Part model, mm, in its own coordinate system. Coordinates: 2 decimals unless noted, no trailing zeros. Loops run counter-clockwise (first coordinate to the right, second up) from the corner with the lowest first, then second, coordinate; pieces in that order, holes last. Notation, with made-up numbers: M 36,25.5 L 58,25.5 A25 ccw 58,46.5 Z; hole C 19.5,70.25 d4. An arc over 180 degrees is marked long. Use a Markdown table: item, result. Add a question column.
1) Wall check: probe 1 along Y at (x, z) = (6.45, 2.75); probe 2 along Y at (x, z) = (5.7, 5); probe 3 along Z at (x, y) = (6.65, -2.5). Give the ranges that are in metal, low to high. Write a range as from..to.
2) Band-saw the part on A-A (z = 9). List the corners of the cut face in (x, y), plus the area to 3 significant figures.
3) Pull direction Y, two halves, no side cores. Call faces 1 (the cylindrical face through (6.089, -6.579, 0.285)), 2 (the flat face through (8, 0, 0)), 3 (the cylindrical face through (4.68, 5.44, 5.57)): released by +Y, released by -Y, zero draft, split by the parting line, or undercut.
4) Pin check, flat tip, straight feed: pin 1 Ø1 at (x, z) = (9, 2) entering from -Y. Stop position of the tip, or through.
from build123d import *

# Parameters (mm, degrees)
BOSS_EXTRUDE1_DEPTH = 11
FILLET1_R           = 1
FILLET2_R           = 1
FILLET3_R           = 0.25


with BuildPart() as part:
    # Sketch1 → Boss-Extrude1 (new body)
    with BuildSketch(Plane.XY):
        with BuildLine():
            Line((6.738137725, -6.88), (4.878137725, -6.88))
            Line((4.878137725, -6.88), (4.531835438, -5.38))
            ThreePointArc((4.531835438, -5.38), (7.034339517, 0), (4.531835438, 5.38))
            Line((4.531835438, 5.38), (4.878137725, 6.88))
            Line((4.878137725, 6.88), (6.738137725, 6.88))
            ThreePointArc((6.738137725, 6.88), (9.63, 0), (6.738137725, -6.88))
        make_face()
    extrude(amount=BOSS_EXTRUDE1_DEPTH)

    # Fillet1
    fillet1_edges = [part.edges().sort_by_distance(p)[0] for p in [
        (4.531835438, -5.38, 5.5),
        (4.531835438, 5.38, 5.5),
    ]]
    fillet(fillet1_edges, radius=FILLET1_R)

    # Fillet2
    fillet2_edges = [part.edges().sort_by_distance(p)[0] for p in [
        (5.808137725, -6.88, 0),
        (5.808137725, -6.88, 11),
        (5.808137725, 6.88, 11),
        (5.808137725, 6.88, 0),
    ]]
    fillet(fillet2_edges, radius=FILLET2_R)

    # Fillet3
    fillet3_edges = [part.edges().sort_by_distance(p)[0] for p in [
        (7.034339517, 0, 0),
        (4.687877266, 5.411310183, 0),
        (7.034339517, 0, 11),
        (4.687877266, -5.411310183, 11),
        (6.738137725, -6.88, 5.5),
        (4.878137725, -6.88, 5.5),
        (9.63, 0, 0),
        (6.738137725, 6.88, 5.5),
        (9.63, 0, 11),
        (7.064336587, 6.544619823, 0.252818297),
        (7.064336587, 6.544619823, 10.747181703),
        (7.064336589, -6.544619821, 10.747181705),
        (7.064336577, -6.544619807, 0.2528183),
        (4.687877266, -5.411310183, 0),
        (4.655934772, -5.914769545, 10.999395357),
        (4.655934772, -5.914769545, 0.000604643),
        (4.815123489, -6.607055355, 10.686578845),
        (4.815123489, -6.607055355, 0.313421155),
        (4.687877266, 5.411310183, 11),
        (4.655934776, 5.914769544, 0.00060465),
        (4.655934776, 5.914769544, 10.99939535),
        (4.878137725, 6.88, 5.5),
        (4.815123489, 6.607055355, 0.313421155),
        (4.815123489, 6.607055355, 10.686578845),
    ]]
    fillet(fillet3_edges, radius=FILLET3_R)


solid = part.part
Entries:
| question | item | result |
|---|---|---|
| 1 | probe 1 | -6.88..-2.81, 2.81..6.88 |
| 1 | probe 2 | -6.88..-4.12, 4.12..6.88 |
| 1 | probe 3 | 0.08..10.92 |
| 2 | outline | M 4.66,-5.95 L 4.83,-6.69 A0.25 ccw 5.08,-6.88 L 6.64,-6.88 A0.25 ccw 6.81,-6.81 A9.63 ccw 6.81,6.81 A0.25 ccw 6.64,6.88 L 5.08,6.88 A0.25 ccw 4.83,6.69 L 4.66,5.95 A1 ccw 4.94,5.01 A7.03 cw 4.94,-5.01 A1 ccw Z |
| 2 | area | 38.5 mm2 |
| 3 | face 1 | released by -Y |
| 3 | face 2 | zero draft |
| 3 | face 3 | undercut |
| 4 | pin 1 | y = -4.53 |
